Answer from the drawing. Dimensions are ordinates in mm from the lowest x, y and z of the part. A direction names the side the tool comes from. Round coordinates to 2 decimals unless told otherwise and drop trailing zeros. Write each loop counter-clockwise with the first axis right and the second up, starting at its lowest first coordinate (ties: lowest second). Pieces come first, ordered by that corner, then holes. Notation, with made-up numbers: (70.5, -23.5) - (129.5, -23.5) arc R25 ccw to (129.5, -8.5) - close; hole circle Ø7 at (3.25, 32.25). An arc over 180 degrees is marked (long way). Answer in a Markdown table with one row per item.
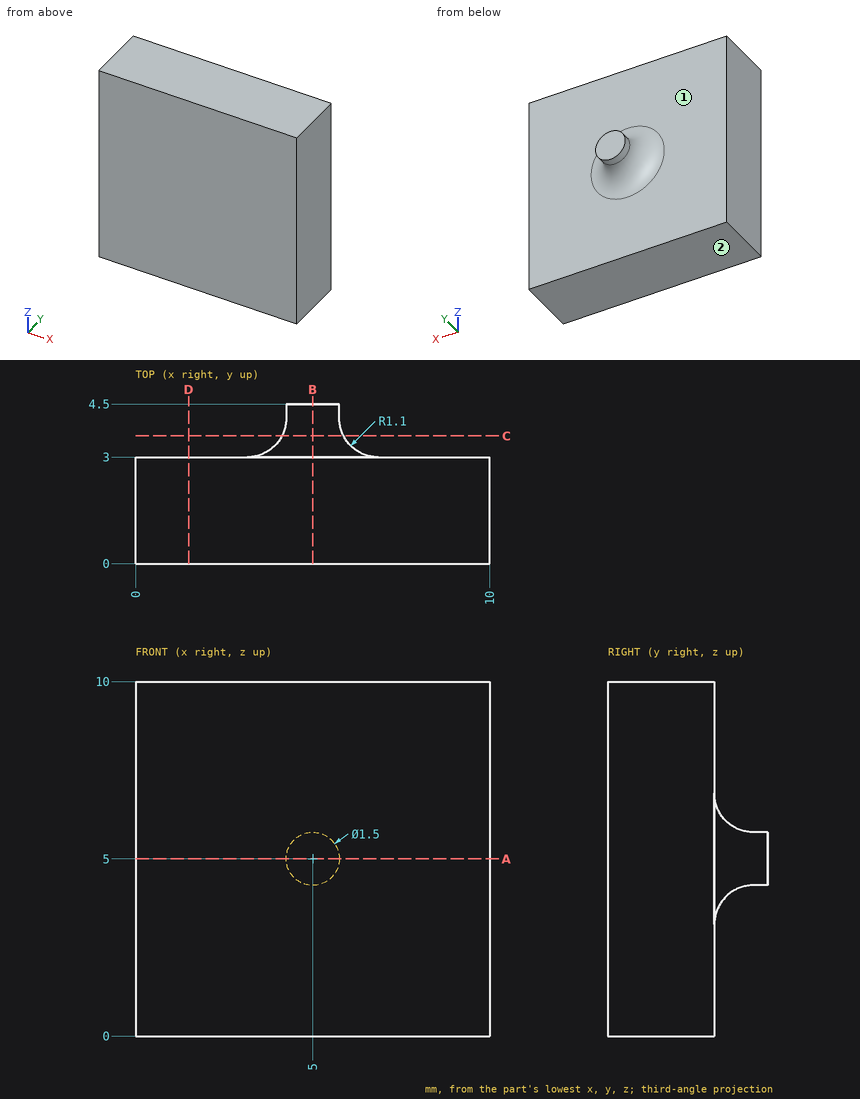
(1) Section B-B (x = 5) is taken. Give the vertices of the cut face in (y, z), and give its area (3 significant figures).
Checked values:
| item | result |
|---|---|
| outline | (0, 0) - (3, 0) - (3, 3.15) arc R1.1 cw to (4.1, 4.25) - (4.5, 4.25) - (4.5, 5.75) - (4.1, 5.75) arc R1.1 cw to (3, 6.85) - (3, 10) - (0, 10) - close |
| area | 32.8 mm2 |
(2) Section D-D (x = 1.5) is taken. Give the vertices of the cut face in (y, z).
Checked values:
| item | result |
|---|---|
| outline | (0, 0) - (3, 0) - (3, 10) - (0, 10) - close |
(3) Section C-C (y = 3.6) is taken. Give the vertices of the cut face in (x, z), and give its area (3 significant figures).
Checked values:
| item | result |
|---|---|
| outline | circle Ø1.74 at (5, 5) |
| area | 2.38 mm2 |
(4) A flat-ended cylindrical pin translates along its axis: pin 1 (2 mm diameter, centred on x = 5.5, y = 3.5, fed in from -Z). Find the tip coordinate at first contact, or state that the pin passes through.
Checked values:
| item | result |
|---|---|
| pin 1 | stops at z = 0 |
(5) Find the intervals of material crossed by line 1 (Y direction, x = 2.25, z = 8); line 2 (Z direction, x = 5, y = 4.1), in increasing order.
Checked values:
| item | result |
|---|---|
| line 1 | y = 0 to 3 |
| line 2 | z = 4.25 to 5.75 |
(6) For the marked faces 1 and 2, determine the directions among +Z, -Z, +X, -X, +Y, -Y from which every point of the face is accessible in a straight line to the end or side of a thin tool.
Checked values:
| item | result |
|---|---|
| face 1 | +Y |
| face 2 | -Z, +X, -X, +Y, -Y |
(7) Section A-A (z = 5) is taken. Give the vertices of the cut face in (x, y).
Checked values:
| item | result |
|---|---|
| outline | (0, 0) - (10, 0) - (10, 3) - (6.85, 3) arc R1.1 cw to (5.75, 4.1) - (5.75, 4.5) - (4.25, 4.5) - (4.25, 4.1) arc R1.1 cw to (3.15, 3) - (0, 3) - close |
